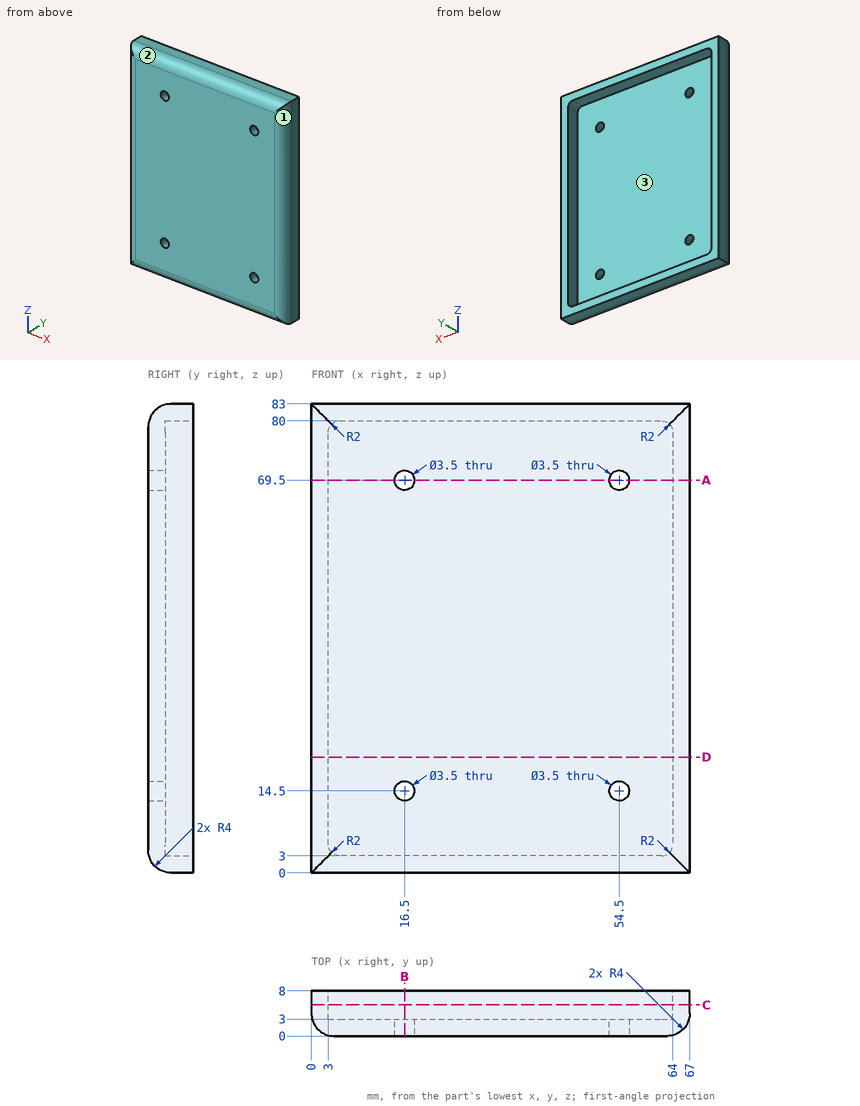
Can you work these out from the drawing? Everything is in mm from the part's minimum corner. Give positions to 0.01 mm unless a question says otherwise; leave off trailing zeros. Order: outer loops, then holes, each group sorted by start corner. A loop starts at its lowest first (then second) coordinate and runs counter-clockwise, first axis right, second up. Notation, with made-up numbers: (78, -8) -> (89, -8) arc R9 cw to (89, 8) -> close; hole circle Ø4 at (86, 86). An arc over 180 degrees is marked (long way). Return JSON: item names as keys, results as strings.
1. For pin 1 Ø4.5 at (x, z) = (54.5, 14.5) entering from +Y, with a flat end and sliding along its axis, tell me the tip position at first contact or that it passes through.
Answer list:
{"pin 1": "stops at y = 3"}
2. I need wall thicknesses on line 1 (X direction, y = 6, z = 14); line 2 (X direction, y = 0.7, z = 14.5); line 3 (Z direction, x = 54.5, y = 1). Which ranges of each line are inside material? Lowest first, please. Write a range as from..to.
Answer list:
{"line 1": "x = 0..3, 64..67", "line 2": "x = 1.74..14.75, 18.25..52.75, 56.25..65.26", "line 3": "z = 1.35..12.75, 16.25..67.75, 71.25..81.65"}
3. Thinking about a two-plate mould opening in X: for the marked faces 1, 2 and 3, which applies, pulls with the +X half, pulls with the -X half, needs draft (parallel to the pull), parting line crosses it, or undercut?
Answer list:
{"face 1": "pulls with the +X half", "face 2": "needs draft", "face 3": "undercut"}
4. Imagine slicing it at A-A on z = 69.5. List the corners of the cut face in (x, y) for me.
Answer list:
{"outline": "(0, 4) arc R4 ccw to (4, 0) -> (14.75, 0) -> (14.75, 3) -> (3, 3) -> (3, 8) -> (0, 8) -> close; (18.25, 0) -> (52.75, 0) -> (52.75, 3) -> (18.25, 3) -> close; (56.25, 0) -> (63, 0) arc R4 ccw to (67, 4) -> (67, 8) -> (64, 8) -> (64, 3) -> (56.25, 3) -> close"}
5. Imagine slicing it at D-D on z = 20.5. List the corners of the cut face in (x, y) for me, then the cut area to 3 significant figures.
Answer list:
{"outline": "(0, 4) arc R4 ccw to (4, 0) -> (63, 0) arc R4 ccw to (67, 4) -> (67, 8) -> (64, 8) -> (64, 3) -> (3, 3) -> (3, 8) -> (0, 8) -> close", "area": "224 mm2"}
6. Imagine slicing it at B-B on x = 16.5. List the corners of the cut face in (y, z) for me.
Answer list:
{"outline": "(0, 4) arc R4 ccw to (4, 0) -> (8, 0) -> (8, 3) -> (3, 3) -> (3, 12.75) -> (0, 12.75) -> close; (0, 16.25) -> (3, 16.25) -> (3, 67.75) -> (0, 67.75) -> close; (0, 71.25) -> (3, 71.25) -> (3, 80) -> (8, 80) -> (8, 83) -> (4, 83) arc R4 ccw to (0, 79) -> close"}
7. Imagine slicing it at C-C on y = 5.5. List the corners of the cut face in (x, z) for me, then the cut area to 3 significant figures.
Answer list:
{"outline": "(0, 0) -> (67, 0) -> (67, 83) -> (0, 83) -> close; hole (3, 5) arc R2 ccw to (5, 3) -> (62, 3) arc R2 ccw to (64, 5) -> (64, 78) arc R2 ccw to (62, 80) -> (5, 80) arc R2 ccw to (3, 78) -> close", "area": "867 mm2"}
